The model under review builds one solid part; all positions refer to its coordinate system, in mm. A direction names the side the tool comes from. Round coordinates to 2 decimals unless told otherwise and drop trailing zeros. Loops run counter-clockwise (first coordinate to the right, second up) from the corner with the lowest first, then second, coordinate; pieces in that order, holes last. Notation, with made-up numbers: (71.25, -30) -> (114.25, -30) arc R25 cw to (114.25, -7) -> close; hole circle Ø2 at (8, 5.25). An arc over 180 degrees is marked (long way). Use a Markdown table: item, result. Add a question column.
1) For faces 1 (the flat face through (0, -12, 8)), 2 (the flat face through (-3, 12, 4)), 3 (the conical face through (0.4, -10.13, 0.36)), list the 3-axis set-ups (+Z, -Z, +X, -X, +Y, -Y) from which the entire face can be reached by the end or side of a thin tool; tool diameter is ignored.
2) Insertion check: pin 1 (4.5 mm diameter, centred on y = 11, z = 5.5, fed in from +X); pin 2 (23 mm diameter, centred on x = 0, y = 0, fed in from +Z); pin 3 (6 mm diameter, centred on y = 36, z = 3.5, fed in from +X). Each pin has a flat end and moves straight along its axis. Give the tip position at first contact, or say it passes through.
3) Wall thickness on probe 1 along X at (y, z) = (18.75, 2.75); probe 2 along X at (y, z) = (21.5, 9); probe 3 along Y at (x, z) = (-30, 6): over which ranges is each line inside the solid? List them lowest first.
4) Consider section B-B on y = 0. Give the boundary of the cut face in (x, z).
5) Consider section A-A on x = 0. Give the boundary of the cut face in (y, z).
6) Mouldability with a two-part tool opening along Y and no side actions: class faces 4 (the cylindrical face through (-29.946, 20.363, 4.93)), 5 (the flat face through (0, 13.5, 4)), 6 (the flat face through (-12, 1, 0)), 7 (the cylindrical face through (47.69, -15.02, 3.94)) as released by +Y, released by -Y, zero draft, split by the parting line, or undercut.
7) Consider section D-D on y = -18.75. State how many separate pieces and enclosed holes the cut face has, plus the area to 3 significant figures.
Autodesk Inventor part; units mm, degrees
ref_plane "YZ Plane" through (0, 0, 0) normal (1, 0, 0) x (0, 1, 0)
ref_plane "XZ Plane" through (0, 0, 0) normal (0, 1, 0) x (-1, 0, 0)
ref_plane "XY Plane" through (0, 0, 0) normal (0, 0, 1) x (1, 0, 0)
sketch "Sketch1" plane through (0, 0, 0) normal (0, 0, 1) x (1, 0, 0)
  circle A0 centre (0, 0) radius 50
  dimension "d0" = 100
extrude "Extrusion1" add sketch "Sketch1" along normal blind 10
sketch "Sketch2" plane through (0, 0, 10) normal (0, 0, 1) x (1, 0, 0)
  arc A0 (-3, 9.5394) -> (3, 9.5394) centre (0, 0) ccw
  line L0 (3, 9.5394) -> (3, 13.5)
  line L1 (3, 13.5) -> (-3, 13.5)
  line L2 (-3, 13.5) -> (-3, 9.5394)
  line L3 (-3, 6.5) -> (3, 13.5) construction
  line L4 (3, 6.5) -> (-3, 13.5) construction
  point P0 (0, 10)
  dimension "d3" = 20
  dimension "d4" = 6
  dimension "d5" = 3.5
extrude "Extrusion2" cut sketch "Sketch2" against normal blind 10
chamfer "Chamfer1" distance 2 angle 45 1 edges at (-50, 0, 10)
sketch "Sketch3" plane through (0, 0, 10) normal (0, 0, 1) x (1, 0, 0)
  circle A0 centre (0, 0) radius 27.5
  dimension "d11" = 55
extrude "Extrusion3" cut sketch "Sketch3" against normal blind 2
chamfer "Chamfer2" distance 0.5 angle 45 2 edges at (0, -10, 0) (0, -10, 8)
sketch "Sketch4" plane through (0, 0, 10) normal (0, 0, 1) x (1, 0, 0)
  line L0 (0, 0) -> (0, 37.5)
  circle A0 centre (0, 37.5) radius 3
  dimension "d17" = 37.5
  dimension "d18" = 6
hole "Hole1" at (0, 37.5, 10) direction (0, 0, -1) diameter 6 end through all
pattern_circular "Circular Pattern1" count 6 over 360 about axis through (0, 0, 10) along (0, 0, -1) of "Hole1"
properties part number "Hub Flange"
Result set:
| question | item | result |
|---|---|---|
| 1 | face 1 | +Z |
| 1 | face 2 | +Z, -Z |
| 1 | face 3 | -Z |
| 2 | pin 1 | x = 49.23 |
| 2 | pin 2 | z = 8 |
| 2 | pin 3 | x = 37.56 |
| 3 | probe 1 | -46.35 to -35.48, -29.48 to 29.48, 35.48 to 46.35 |
| 3 | probe 2 | -44.03 to -33.67, -31.28 to -17.15, 17.15 to 31.28, 33.67 to 44.03 |
| 3 | probe 3 | -40 to -20.44, -17.06 to 17.06, 20.44 to 40 |
| 4 | outline | (-50, 0) -> (-10.5, 0) -> (-10, 0.5) -> (-10, 7.5) -> (-10.5, 8) -> (-27.5, 8) -> (-27.5, 10) -> (-48, 10) -> (-50, 8) -> close; (10, 0.5) -> (10.5, 0) -> (50, 0) -> (50, 8) -> (48, 10) -> (27.5, 10) -> (27.5, 8) -> (10.5, 8) -> (10, 7.5) -> close |
| 5 | outline | (-50, 0) -> (-40.5, 0) -> (-40.5, 10) -> (-48, 10) -> (-50, 8) -> close; (-34.5, 0) -> (-10.5, 0) -> (-10, 0.5) -> (-10, 7.5) -> (-10.5, 8) -> (-27.5, 8) -> (-27.5, 10) -> (-34.5, 10) -> close; (13.5, 0) -> (34.5, 0) -> (34.5, 10) -> (27.5, 10) -> (27.5, 8) -> (13.5, 8) -> close; (40.5, 0) -> (50, 0) -> (50, 8) -> (48, 10) -> (40.5, 10) -> close |
| 6 | face 4 | undercut |
| 6 | face 5 | undercut |
| 6 | face 6 | zero draft |
| 6 | face 7 | split by the parting line |
| 7 | separate pieces | 3 |
| 7 | enclosed holes | 0 |
| 7 | area | 722 mm2 |
